Check sheet for the modelled part. Datum: model origin and axes. Units: mm. Face numbers are marked on the shaded views. A direction names the side the tool comes from. Give positions to 0.01 mm unless a question says otherwise; leave off trailing zeros. Order: outer loops, then holes, each group sorted by start corner. A loop starts at its lowest first (then second) coordinate and runs counter-clockwise, first axis right, second up.
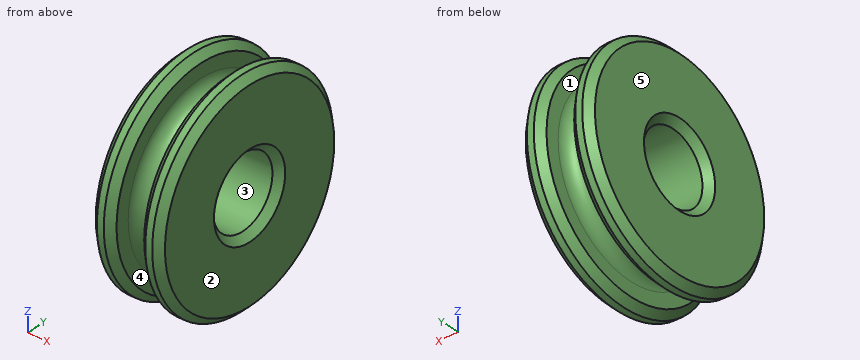
```python
from build123d import *

# Parameters (mm, degrees)
CHANFREIN1_SIZE = 1


with BuildPart() as part:
    # Esquisse1 → Révolution1 (revolve)
    with BuildSketch(Plane(origin=(0, 0, 0), x_dir=(0, 1, 0), z_dir=(0, 0, 1)), mode=Mode.PRIVATE) as r_volution1_sk:
        with BuildLine():
            Line((5.1, 10), (5.1, 0))
            Line((5.1, 0), (15.5, 0))
            Line((15.5, 0), (15.5, 3))
            Line((15.5, 3), (12.5, 3))
            ThreePointArc((12.5, 3), (10.5, 5), (12.5, 7))
            Line((12.5, 7), (15.5, 7))
            Line((15.5, 7), (15.5, 10))
            Line((15.5, 10), (5.1, 10))
        make_face()
    revolve(r_volution1_sk.sketch.rotate(Axis((0, 0, 0), (-1, 0, 0)), 90), axis=Axis((0, 0, 0), (-1, 0, 0)))

    # Chanfrein1
    chanfrein1_edges = [part.edges().sort_by_distance(p)[0] for p in [
        (-10, 0, 15.5),
        (-7, 0, 15.5),
        (-3, 0, 15.5),
        (0, 0, 15.5),
        (0, 0, 5.1),
        (-10, 0, 5.1),
    ]]
    chamfer(chanfrein1_edges, length=CHANFREIN1_SIZE)


solid = part.part
```
(1) Material ranges on L1, parallel to X at y = -12, z = -3.5; L2, parallel to Y at x = -8, z = 2; L3, parallel to Y at x = -5.25, z = 0, recorded low to high.
Response values:
L1: x = -10 to -7, -3 to 0
L2: y = -15.37 to -4.69, 4.69 to 15.37
L3: y = -10.52 to -5.1, 5.1 to 10.52
(2) Set-up check for the marked faces 1 and 2: record each of +Z, -Z, +X, -X, +Y, -Y from which the full face is reachable in a straight line by a thin tool's end or side.
Response values:
face 1: none
face 2: +Z, -Z, +X, +Y, -Y
(3) Release check for a two-part mould opening along X. For the marked faces 3, 4 and 5 record: released by +X, released by -X, zero draft, split by the parting line, or undercut.
Response values:
face 3: zero draft
face 4: undercut
face 5: released by -X
(4) Cross-section at A-A on y = 0. Enter the section's corners in (x, z).
Response values:
outline: (-10, -14.5) - (-9, -15.5) - (-8, -15.5) - (-7, -14.5) - (-7, -12.5) arc R2 cw to (-3, -12.5) - (-3, -14.5) - (-2, -15.5) - (-1, -15.5) - (0, -14.5) - (0, -6.1) - (-1, -5.1) - (-9, -5.1) - (-10, -6.1) - close; (-10, 6.1) - (-9, 5.1) - (-1, 5.1) - (0, 6.1) - (0, 14.5) - (-1, 15.5) - (-2, 15.5) - (-3, 14.5) - (-3, 12.5) arc R2 cw to (-7, 12.5) - (-7, 14.5) - (-8, 15.5) - (-9, 15.5) - (-10, 14.5) - close
(5) Gauge pin test, flat ends, axial feed: pin 1 Ø4 at (x, z) = (-2, -11) entering from -Y; pin 2 Ø4 at (x, y) = (-3, 2) entering from -Z; pin 3 Ø1.5 at (x, z) = (-2.5, 2.5) entering from -Y. Record the tip position at first contact, or that the pin passes through.
Response values:
pin 1: stops at y = -12.62
pin 2: stops at z = -15.5
pin 3: stops at y = -15.38
